CAD build for the part. Positions are in the model's coordinates, mm. A direction names the side the tool comes from. Round coordinates to 2 decimals unless told otherwise and drop trailing zeros. Loops run counter-clockwise (first coordinate to the right, second up) from the corner with the lowest first, then second, coordinate; pieces in that order, holes last. Notation, with made-up numbers: M 89.5,6.25 L 99.5,6.25 A21 cw 99.5,22.25 Z; hole C 83.5,-27.75 d1. An arc over 180 degrees is marked long. Use a Markdown table: item, result. Add a question column.
(1) Wall check: L1, parallel to Z at x = -2.5, y = -0.75; L2, parallel to Z at x = -1.5, y = 0.5; L3, parallel to Y at x = -0.25, z = -3.25. Give the ranges that are in metal, low to high.
(2) Band-saw the part on B-B, the plane z = -6. Write the cut outline in (x, y).
(3) Which spindle directions (+Z, -Z, +X, -X, +Y, -Y) get a long thin tool onto all of the face, cutting with end or side? Do faces 1 (the face through (0, 0, 1)), 2 (the face through (-1.5, 0.07, -7.89)). Say none if no direction does.
(4) Flat gauge pins, fed straight in: P1, Ø2, axis at x = 1.5, z = -11.5, coming from the -Y side; P2, Ø3, axis at x = 0.5, z = -13, coming from the -Y side; P3, Ø2, axis at x = -2.5, y = -1.5, coming from the -Z side. Where does each tip first touch, or does it go through?
(5) Band-saw the part on A-A, the plane y = 0. Write the cut outline in (x, z), and give its area (3 significant figures).
(6) Band-saw the part on C-C, the plane y = -1. Write the cut outline in (x, z).
from build123d import *

# Parameters (mm, degrees)
SKETCH_1_R      = 1.5
EXTRUDE_1_DEPTH = 16
SKETCH_2_R      = 2
EXTRUDE_2_DEPTH = 0.5
EXTRUDE_3_DEPTH = 0.5


with BuildPart() as part:
    # 草圖1 → 填料-伸長1 (new body)
    with BuildSketch(Plane.XY):
        Circle(SKETCH_1_R)
    extrude(amount=-EXTRUDE_1_DEPTH)

    # 草圖2 → 填料-伸長2 (add)
    with BuildSketch(Plane.XY):
        Circle(SKETCH_2_R)
    extrude(amount=EXTRUDE_2_DEPTH)

    # 草圖3 → 填料-伸長3 (add)
    with BuildSketch(Plane.XY.offset(0.5)):
        with BuildLine():
            Line((-0.91486326, 2.834533474), (-2.970311666, -0.220914932))
            ThreePointArc((-2.970311666, -0.220914932), (-3.045533313, -0.400920314), (-3.046143975, -0.59600968))
            ThreePointArc((-3.046143975, -0.59600968), (0, -3.103904099), (3.046143975, -0.59600968))
            ThreePointArc((3.046143975, -0.59600968), (3.045533313, -0.400920314), (2.970311666, -0.220914932))
            Line((2.970311666, -0.220914932), (0.91486326, 2.834533474))
            ThreePointArc((0.91486326, 2.834533474), (0.776482443, 2.972050685), (0.59600968, 3.046143975))
            ThreePointArc((0.59600968, 3.046143975), (0.299400973, 3.089430321), (0, 3.103904099))
            ThreePointArc((0, 3.103904099), (-0.299400973, 3.089430321), (-0.59600968, 3.046143975))
            ThreePointArc((-0.59600968, 3.046143975), (-0.776482443, 2.972050685), (-0.91486326, 2.834533474))
        make_face()
    extrude(amount=EXTRUDE_3_DEPTH)


solid = part.part
Return value:
| question | item | result |
|---|---|---|
| 1 | L1 | 0.5 to 1 |
| 1 | L2 | 0 to 1 |
| 1 | L3 | -1.48 to 1.48 |
| 2 | outline | C 0,0 d3 |
| 3 | face 1 | +Z, +X, -X, +Y, -Y |
| 3 | face 2 | -Z |
| 4 | P1 | y = -1.41 |
| 4 | P2 | y = -1.5 |
| 4 | P3 | z = 0 |
| 5 | outline | M -2.82,0.5 L -2,0.5 L -2,0 L -1.5,0 L -1.5,-16 L 1.5,-16 L 1.5,0 L 2,0 L 2,0.5 L 2.82,0.5 L 2.82,1 L -2.82,1 Z |
| 5 | area | 52.8 mm^2 |
| 6 | outline | M -2.94,0.5 L -1.73,0.5 L -1.73,0 L -1.12,0 L -1.12,-16 L 1.12,-16 L 1.12,0 L 1.73,0 L 1.73,0.5 L 2.94,0.5 L 2.94,1 L -2.94,1 Z |
